Autodesk Inventor part; units mm, degrees
ref_plane "YZ Plane" through (0, 0, 0) normal (1, 0, 0) x (0, 1, 0)
ref_plane "XZ Plane" through (0, 0, 0) normal (0, 1, 0) x (-1, 0, 0)
ref_plane "XY Plane" through (0, 0, 0) normal (0, 0, 1) x (1, 0, 0)
sketch "Sketch1" plane through (0, 0, 0) normal (0, 1, 0) x (-1, 0, 0)
  line L0 (0, 0) -> (70.6, 0)
  line L1 (70.6, 0) -> (70.6, -11)
  line L2 (70.6, -11) -> (0, -11)
  line L3 (0, -11) -> (0, 0)
  dimension "d0" = 70.6
  dimension "d1" = 11
extrude "Extrusion1" add sketch "Sketch1" along normal blind 11
sketch "Sketch2" plane through (-70.6, 0, 0) normal (0, 0, 1) x (1, 0, 0)
  circle A0 centre (6.3, 5.5) radius 3.15
  circle A1 centre (64.3, 5.5) radius 3.15
  line L0 (6.3, 5.5) -> (64.3, 5.5) construction
  line L1 (0, 11) -> (70.6, 11) construction
  line L2 (0, 0) -> (0, 11) construction
  circle A2 centre (6.3, 5.5) radius 4.15
  circle A3 centre (64.3, 5.5) radius 4.15
  point P0 (70.6, 0)
  dimension "d4" = 5.5
  dimension "d5" = 58
  dimension "d6" = 6.3
  dimension "d7" = 6.3
  dimension "d8" = 1
extrude "Extrusion2" add sketch "Sketch2" along normal blind 5
equation "\"d0\" = carriage_support_length"
equation "\"d1\" = carriage_support_width"
equation "\"d2\" = carriage_support_height"
equation "\"d4\" = 0.5 * carriage_support_height"
equation "\"d5\" = carriage_rod_dist"
equation "\"d6\" = 0.5 * carriage_support_length - 0.5 * carriage_rod_dist"
equation "\"d7\" = carriage_rod_diameter + rod_tolerance"
equation "\"carriage_rod_diameter\" = 6"
equation "\"rod_tolerance\" = 0.3"
equation "\"carriage_support_length\" = 70.6"
equation "\"carriage_support_width\" = 11"
equation "\"carriage_support_height\" = 11"
equation "\"carriage_rod_dist\" = 58"
properties part number "carriage_support"
Geometry check sheet. Reference: the model listing, model coordinates, mm. A direction names the side the tool comes from. Give positions to 0.01 mm unless a question says otherwise; leave off trailing zeros. Write each loop counter-clockwise with the first axis right and the second up, starting at its lowest first coordinate (ties: lowest second). Pieces come first, ordered by that corner, then holes. Notation, with made-up numbers: (-18, 8) - (-3, 8) arc R18 cw to (-3, 17) - close; hole circle Ø5 at (21, 52). An arc over 180 degrees is marked (long way). Put each result on its own line as item: value.
1. Draft check along X on faces 3 (the flat face through (-70.6, 5, -5)), 4 (the flat face through (-36, 5, -11)), 5 (the flat face through (-64, 5, 0)). Enter one of: +X half, -X half, draft (parallel to the pull), parting line (faces both ways), or undercut.
Ans:
face 3: -X half
face 4: draft
face 5: undercut
2. Sectioned sample at B-B, the plane z = 2.5. Enter the section's corners in (x, y), plus the area to 3 significant figures.
Ans:
outline: circle Ø8.3 at (-64.3, 5.5); circle Ø8.3 at (-6.3, 5.5); hole circle Ø6.3 at (-64.3, 5.5); hole circle Ø6.3 at (-6.3, 5.5)
area: 45.9 mm²
3. Go/stop test with flat-tipped pins: pin 1 (1.9 mm diameter, centred on x = -7.5, y = 6, fed in from +Z); pin 2 (1 mm diameter, centred on y = 6.5, z = 1.5, fed in from +X); pin 3 (5 mm diameter, centred on x = -63.5, y = 4.5, fed in from +Z). Record where each tip stops, or that it passes through.
Ans:
pin 1: stops at z = 0
pin 2: stops at x = -2.18
pin 3: stops at z = 5
4. Sectioned sample at D-D, the plane y = 10.25. Enter the section's corners in (x, z), plus the area to 3 significant figures.
Ans:
outline: (-70.6, -11) - (0, -11) - (0, 0) - (-70.6, 0) - close
area: 777 mm²
5. Sectioned sample at C-C, the plane x = -6.3. Enter the section's corners in (y, z).
Ans:
outline: (0, -11) - (11, -11) - (11, 0) - (9.65, 0) - (9.65, 5) - (8.65, 5) - (8.65, 0) - (2.35, 0) - (2.35, 5) - (1.35, 5) - (1.35, 0) - (0, 0) - close
6. Set-up check for faces 1 (the cylindrical face through (-68.446, 5.318, 2.465)), 2 (the flat face through (-35, 0, -5)): record each of +Z, -Z, +X, -X, +Y, -Y from which the full face is reachable in a straight line by a thin tool's end or side.
Ans:
face 1: +Z
face 2: +Z, -Z, +X, -X, -Y
7. Thickness scan on line 1 (Y direction, x = -6.3, z = 3.65); line 2 (X direction, y = 6, z = 2.75); line 3 (Z direction, x = -67, y = 5). Record the ranges inside material, lowest first.
Ans:
line 1: y = 1.35 to 2.35, 8.65 to 9.65
line 2: x = -68.42 to -67.41, -61.19 to -60.18, -10.42 to -9.41, -3.19 to -2.18
line 3: z = -11 to 0
8. Sectioned sample at A-A, the plane y = 5.5. Enter the section's corners in (x, z), plus the area to 3 significant figures.
Ans:
outline: (-70.6, -11) - (0, -11) - (0, 0) - (-2.15, 0) - (-2.15, 5) - (-3.15, 5) - (-3.15, 0) - (-9.45, 0) - (-9.45, 5) - (-10.45, 5) - (-10.45, 0) - (-60.15, 0) - (-60.15, 5) - (-61.15, 5) - (-61.15, 0) - (-67.45, 0) - (-67.45, 5) - (-68.45, 5) - (-68.45, 0) - (-70.6, 0) - close
area: 797 mm²
